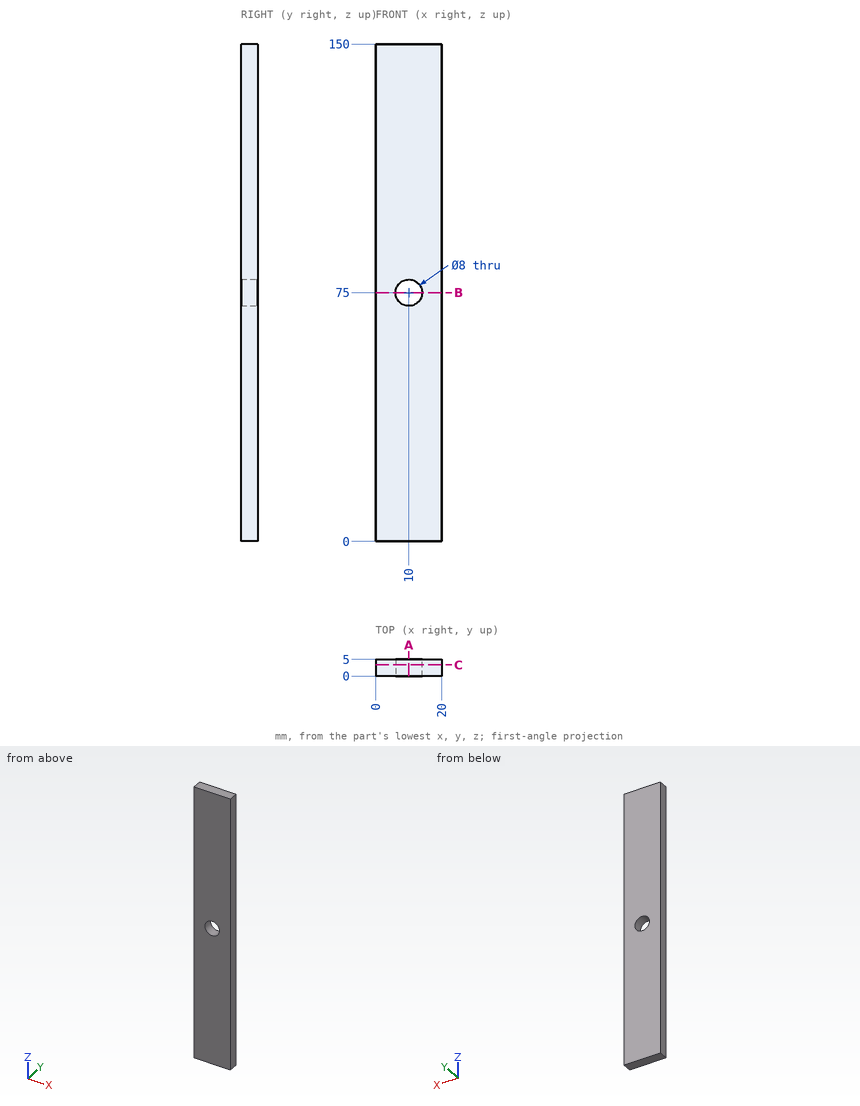
Input: dimensioned drawing with shaded views. Units: mm. Origin: part minimum x, y, z. Round coordinates to 2 decimals unless told otherwise and drop trailing zeros. Loops run counter-clockwise (first coordinate to the right, second up) from the corner with the lowest first, then second, coordinate; pieces in that order, holes last. Notation, with made-up numbers: (-29, 85.25) -> (16, 85.25) arc R23 ccw to (16, 116.25) -> close; hole circle Ø7 at (-14.75, 75). An arc over 180 degrees is marked (long way). Answer as a JSON object with one key per item and string values. Group by question number.
Q1. Section query A-A (x = 10). Output: boundary loops of the cut face in (y, z), plus the area to 3 significant figures.
Q2. Ray query, line 1 (Z direction, x = 10, y = 3.55); line 2 (Z direction, x = 6.5, y = 2.15). Return the intervals inside material, ascending. Write a range as from..to.
Q3. Section query B-B (z = 75). Output: boundary loops of the cut face in (x, y).
Q4. Section query C-C (y = 3.35). Output: boundary loops of the cut face in (x, z).
Completed:
{
 "1": {"outline": "(0, 0) -> (5, 0) -> (5, 71) -> (0, 71) -> close; (0, 79) -> (5, 79) -> (5, 150) -> (0, 150) -> close", "area": "710 mm²"},
 "2": {"line 1": "0..71, 79..150", "line 2": "0..73.06, 76.94..150"},
 "3": {"outline": "(0, 0) -> (6, 0) -> (6, 5) -> (0, 5) -> close; (14, 0) -> (20, 0) -> (20, 5) -> (14, 5) -> close"},
 "4": {"outline": "(0, 0) -> (20, 0) -> (20, 150) -> (0, 150) -> close; hole circle Ø8 at (10, 75)"}
}
